CAD build for the part. Positions are in the model's coordinates, mm. A direction names the side the tool comes from. Round coordinates to 2 decimals unless told otherwise and drop trailing zeros. Order: outer loops, then holes, each group sorted by start corner. A loop starts at its lowest first (then second) coordinate and runs counter-clockwise, first axis right, second up. Notation, with made-up numbers: M 64,38.5 L 107,38.5 A25 ccw 107,72.5 Z; hole C 17.5,-34 d7. An arc over 180 degrees is marked long. Answer as a JSON object with one key per item and string values.
```python
from build123d import *

# Parameters (mm, degrees)
F1_DEPTH = 15
F2_R     = 2
F3_R     = 5.875
F4_DEPTH = 2.5
F5_R     = 3
F7_D     = 2


with BuildPart() as f1:
    # F0 (on Top) → F1 (new body)
    with BuildSketch(Plane.XY):
        with BuildLine():
            ThreePointArc((-10.3596491228, 1.7110435565), (-10.0908840346, 0.8742164411), (-10, 0))
            ThreePointArc((-10, 0), (-10.0908840346, -0.8742164411), (-10.3596491228, -1.7110435565))
            ThreePointArc((-10.3596491228, -1.7110435565), (-10.1258015969, -2.778154427), (-9.7823464912, -3.8151929343))
            ThreePointArc((-9.7823464912, -3.8151929343), (-8.7380543651, -2.0332437921), (-8.375, 0))
            ThreePointArc((-8.375, 0), (-8.7380543651, 2.0332437921), (-9.7823464912, 3.8151929343))
            ThreePointArc((-9.7823464912, 3.8151929343), (-10.1258015969, 2.778154427), (-10.3596491228, 1.7110435565))
        make_face()
        with BuildLine():
            ThreePointArc((-10.3596491228, -1.7110435565), (-18.5, 0), (-10.3596491228, 1.7110435565))
            ThreePointArc((-10.3596491228, 1.7110435565), (-10.1258015969, 2.778154427), (-9.7823464912, 3.8151929343))
            ThreePointArc((-9.7823464912, 3.8151929343), (-20.125, 0), (-9.7823464912, -3.8151929343))
            ThreePointArc((-9.7823464912, -3.8151929343), (-10.1258015969, -2.778154427), (-10.3596491228, -1.7110435565))
        make_face()
        with BuildLine():
            ThreePointArc((7.4246212025, 7.4246212025), (-2.1556229355, 10.2763461288), (-9.7823464912, 3.8151929343))
            ThreePointArc((-9.7823464912, 3.8151929343), (-8.7380543651, 2.0332437921), (-8.375, 0))
            ThreePointArc((-8.375, 0), (-3.2049737461, 7.7374910848), (5.9220192924, 5.9220192924))
            Line((5.9220192924, 5.9220192924), (7.4246212025, 7.4246212025))
        make_face()
        with BuildLine():
            ThreePointArc((-8.375, 0), (-8.7380543651, -2.0332437921), (-9.7823464912, -3.8151929343))
            ThreePointArc((-9.7823464912, -3.8151929343), (-2.1556229355, -10.2763461288), (7.4246212025, -7.4246212025))
            Line((7.4246212025, -7.4246212025), (5.9220192924, -5.9220192924))
            ThreePointArc((5.9220192924, -5.9220192924), (-3.2049737461, -7.7374910848), (-8.375, 0))
        make_face()
    extrude(amount=F1_DEPTH)

    # F2
    f2_edges = [f1.edges().sort_by_distance(p)[0] for p in [
        (5.922019, 5.922019, 7.5),
        (5.922019, -5.922019, 7.5),
    ]]
    fillet(f2_edges, radius=F2_R)

    # F3 (on face) → F4 (join)
    with BuildSketch(Plane.XY.offset(15)):
        with Locations((-14.25, 0)):
            Circle(F3_R)
    extrude(amount=-F4_DEPTH)

    # F5
    f5_edges = [f1.edges().sort_by_distance(p)[0] for p in [
        (-9.782346, 3.815193, 7.5),
        (-9.782346, -3.815193, 7.5),
    ]]
    fillet(f5_edges, radius=F5_R)

    # F7 (through all)
    with Locations(Plane.XY.offset(15)):
        with Locations((-14.25, 0)):
            Hole(F7_D / 2)


solid = f1.part
```
Item 1: Saw through at B-B on y = -0.5. List the corners of the cut face in (x, z).
Worked answers:
{"outline": "M -20.1,0 L -18.47,0 L -18.47,12.5 L -15.12,12.5 L -15.12,15 L -20.1,15 Z; M -13.38,12.5 L -10.03,12.5 L -10.03,0 L -8.36,0 L -8.36,15 L -13.38,15 Z"}
Item 2: Wall check: line 1 along Y through (x, z) = (-14.25, 8) (3 decimals); line 2 along X through (y, z) = (-7.5, 7.5); line 3 along Y through (x, z) = (-1.5, 11.75). Give the ranges that are in metal, low to high. Write a range as [from, to].
Worked answers:
{"line 1": "y = [-5.875, -4.25], [4.25, 5.875]", "line 2": "x = [-7.35, -3.73], [3.73, 7.35]", "line 3": "y = [-10.39, -8.24], [8.24, 10.39]"}
Item 3: Two-plate mould, pull along Y, no slides. Class faces 1 (the flat face through (-8.5, 0.8, 0)), 2 (the cylindrical face through (-15.204, 0.3, 13.733)), 3 (the cylindrical face through (-0.591, 10.483, 7.395)): released by +Y, released by -Y, zero draft, split by the parting line, or undercut.
Worked answers:
{"face 1": "zero draft", "face 2": "undercut", "face 3": "released by +Y"}
Item 4: 3-axis set-ups, long thin cutter, end or side, ignore diameter. For faces 4 (the flat face through (-13, -1, 12.5)), 5 (the cylindrical face through (-0.841, -10.466, 7.395)), 6 (the cylindrical face through (5.997, -6.624, 7.605)): which of +Z, -Z, +X, -X, +Y, -Y reach the whole face in a straight line?
Worked answers:
{"face 4": "-Z", "face 5": "+Z, -Z, -Y", "face 6": "+Z, -Z"}
Item 5: Saw through at C-C on x = -14.25. List the corners of the cut face in (y, z) (3 decimals), and give its area (3 significant figures).
Worked answers:
{"outline": "M -5.875,0 L -4.25,0 L -4.25,12.5 L -1,12.5 L -1,15 L -5.875,15 Z; M 1,12.5 L 4.25,12.5 L 4.25,0 L 5.875,0 L 5.875,15 L 1,15 Z", "area": "65.0 mm2"}
Item 6: Drop flat-ended pins along their axis: pin 1 Ø8 at (x, z) = (-13, 10) entering from +Y (3 decimals); pin 2 Ø2.5 at (x, y) = (-12.5, -2) entering from -Z; pin 3 Ø1 at (x, z) = (-13, 3.5) entering from +Y. Give the stop position or say it passes through.
Worked answers:
{"pin 1": "stops at y = 5.875", "pin 2": "stops at z = 12.5", "pin 3": "stops at y = 5.83"}
Item 7: Saw through at A-A on x = 0. List the corners of the cut face in (y, z) (3 decimals), and give its area (4 significant figures).
Worked answers:
{"outline": "M -10.5,0 L -8.375,0 L -8.375,15 L -10.5,15 Z; M 8.375,0 L 10.5,0 L 10.5,15 L 8.375,15 Z", "area": "63.75 mm2"}
Item 8: Saw through at D-D on x = -17.75. List the corners of the cut face in (y, z), and give its area (3 significant figures).
Worked answers:
{"outline": "M -4.72,0 L -2.41,0 L -2.41,12.5 L 2.41,12.5 L 2.41,0 L 4.72,0 L 4.72,15 L -4.72,15 Z", "area": "81.3 mm2"}
